Autodesk Inventor part; units mm, degrees
ref_plane "YZ Plane" through (0, 0, 0) normal (1, 0, 0) x (0, 1, 0)
ref_plane "XZ Plane" through (0, 0, 0) normal (0, 1, 0) x (-1, 0, 0)
ref_plane "XY Plane" through (0, 0, 0) normal (0, 0, 1) x (1, 0, 0)
sketch "Эскиз1" plane through (0, 0, 0) normal (0, 1, 0) x (-1, 0, 0)
  circle A0 centre (0, 0) radius 6.95
  circle A1 centre (0, 0) radius 7.95
  line L0 (0, 0) -> (6.3439, 4.7913)
  line L1 (0, 0) -> (6.3439, -4.7913)
  point P0 (5.546, -4.1887)
  point P1 (5.546, 4.1887)
  dimension "d0" = 13.9
  dimension "d1" = 15.9
extrude "Выдавливание1" add sketch "Эскиз1" along normal blind 30 contours A0 L1 A1 L0 picked at (-7.4629, 1.2262)
sketch "Эскиз2" plane through (0, 30, 0) normal (0, 1, 0) x (1, 0, 0)
  arc A0 (-5.546, -4.1887) -> (-6.4386, -3.6588) centre (-8.2473, -7.7226) ccw
  arc A1 (-6.4386, -3.6588) -> (-7.5956, -5.4645) centre (-6.873, -4.654) ccw
  line L0 (-7.5956, -5.4645) -> (-6.9243, -4.6101)
  arc A2 (-6.3454, -4.7768) -> (-6.9243, -4.6101) centre (-6.7137, -4.9672) ccw
  line L1 (-5.546, -4.1887) -> (-6.3439, -4.7913)
  line L2 (-6.3439, -4.7913) -> (-5.546, -4.1887)
  line L3 (-6.3439, -4.7913) -> (-6.3454, -4.7768)
  line L4 (-0.0151, 0) -> (-3.489, 0)
  arc A3 (-6.4386, 3.6588) -> (-5.546, 4.1887) centre (-8.2473, 7.7226) ccw
  arc A4 (-6.9243, 4.6101) -> (-6.3454, 4.7768) centre (-6.7137, 4.9672) ccw
  line L5 (-5.546, 4.1887) -> (-6.3439, 4.7913)
  line L6 (-6.3439, 4.7913) -> (-5.546, 4.1887)
  line L7 (-6.3439, 4.7913) -> (-6.3454, 4.7768)
  arc A5 (-7.5956, 5.4645) -> (-6.4386, 3.6588) centre (-6.873, 4.654) ccw
  line L8 (-7.5956, 5.4645) -> (-6.9243, 4.6101)
  point P0 (-5.546, 4.1887)
  point P1 (-6.3439, -4.7913)
  point P2 (-5.3694, -4.0591)
  point P3 (-6.3439, 4.7913)
  point P4 (-5.3694, 4.0591)
  point P5 (-6.3439, 4.7913)
  dimension "d25" = 1.0859
sketch "Эскиз3" plane through (0, 30, 0) normal (0, 1, 0) x (1, 0, 0)
  arc A0 (-6.3439, -4.7913) -> (-6.3439, 4.7913) centre (0, 0) ccw
  line L0 (11.5, -6.95) -> (11.5, 6.95)
  arc A1 (-5.546, -4.1887) -> (-5.546, 4.1887) centre (0, 0) ccw
  line L1 (0, -7.95) -> (0, -6.95)
  line L2 (0, 6.95) -> (0, 7.95)
  line L3 (11.5, 6.95) -> (11.5, 10.95)
  line L4 (11.5, -6.95) -> (11.5, -10.95)
  line L5 (0, 3.45) -> (0, 7.95)
  line L6 (11.5, -10.95) -> (0, -10.95)
  line L7 (0, -10.95) -> (0, -7.95)
  line L8 (11.5, 10.95) -> (0, 10.95)
  line L9 (0, 10.95) -> (0, 7.95)
  arc A2 (0, -6.95) -> (0, 6.95) centre (0, 0) ccw
  dimension "d13" = 4
  dimension "d14" = 4
  dimension "d22" = 21.9
  dimension "d23" = 4
extrude "Выдавливание3" add sketch "Эскиз3" against normal blind 30
ref_plane "РабПлоскость1" through (11.5, 20, 4.95) normal (1, 0, 0) x (0, 0, -1)
sketch "Эскиз4" plane through (11.5, 20, 4.95) normal (1, 0, 0) x (0, 0, -1)
  line L0 (4.95, -20) -> (4.95, 10)
  line L1 (1, 10) -> (8.9, 10)
  circle A0 centre (4.95, -12) radius 5
  line L2 (14.4, -20) -> (-4.5, -20)
  circle A1 centre (4.95, 2) radius 5
  line L3 (-4.5, 10) -> (14.4, 10)
  point P0 (7.3306, 10)
  point P1 (2.5694, 10)
  point P2 (4.95, 10)
  dimension "d15" = 10
  dimension "d16" = 8
  dimension "d17" = 10
  dimension "d18" = 8
extrude "Выдавливание4" cut sketch "Эскиз4" against normal blind 2
extrude "Выдавливание5" add sketch "Эскиз2" against normal blind 30
sketch "Эскиз5" plane through (0, 30, 0) normal (0, 1, 0) x (1, 0, 0)
  arc A0 (0, 7.95) -> (-6.3439, 4.7913) centre (0, 0) ccw
  line L0 (-6.3439, 4.7913) -> (-6.3454, 4.7768)
  arc A1 (-6.9243, 4.6101) -> (-6.3454, 4.7768) centre (-6.7137, 4.9672) ccw
  line L1 (-6.9243, 4.6101) -> (-7.5956, 5.4645)
  arc A2 (-7.5956, 5.4645) -> (-6.4386, 3.6588) centre (-6.873, 4.654) ccw
  arc A3 (-6.4386, 3.6588) -> (-5.546, 4.1887) centre (-8.2473, 7.7226) ccw
  arc A4 (-5.546, -4.1887) -> (-5.546, 4.1887) centre (0, 0) ccw
  arc A5 (-5.546, -4.1887) -> (-6.4386, -3.6588) centre (-8.2473, -7.7226) ccw
  arc A6 (-6.4386, -3.6588) -> (-7.5956, -5.4645) centre (-6.873, -4.654) ccw
  line L2 (-7.5956, -5.4645) -> (-6.9243, -4.6101)
  arc A7 (-6.3454, -4.7768) -> (-6.9243, -4.6101) centre (-6.7137, -4.9672) ccw
  line L3 (-6.3454, -4.7768) -> (-6.3439, -4.7913)
  arc A8 (-6.3439, -4.7913) -> (0, -7.95) centre (0, 0) ccw
  line L4 (0, -7.95) -> (0, -10.95)
  line L5 (0, -10.95) -> (11.5, -10.95)
  line L6 (11.5, -10.95) -> (11.5, 10.95)
  line L7 (11.5, 10.95) -> (0, 10.95)
  line L8 (0, 10.95) -> (0, 7.95)
  line L9 (0, 6.95) -> (0, 7.95)
  line L10 (0, -6.95) -> (0, -7.95)
extrude "Выдавливание6" [suppressed]
sketch "Эскиз6" plane through (11.5, 30, 10.95) normal (1, 0, 0) x (0, 0, -1)
  arc A0 (15.95, -22) -> (15.95, -22) centre (10.95, -22) ccw
  arc A1 (15.95, -8) -> (15.95, -8) centre (10.95, -8) ccw
  point P0 (10.95, -30)
extrude "Выдавливание7" [suppressed]
properties part number "крепление маркера 14мм"
The listing builds one solid part. Answer for the finished solid, in the listing's coordinates (mm). A direction names the side the tool comes from. Coordinates: 2 decimals unless noted, no trailing zeros. Loops run counter-clockwise (first coordinate to the right, second up) from the corner with the lowest first, then second, coordinate; pieces in that order, holes last. Notation, with made-up numbers: M -28.75,59 L 23.25,59 A18 ccw 23.25,81 Z; hole C 30,27.25 d11. An arc over 180 degrees is marked long. Answer as CSV lines item,"result". Start each with the question number.
(1) Find the intervals of material crossed by L1, parallel to Y at x = 10.5, z = 0; L2, parallel to Z at x = 10.55, y = 22; L3, parallel to X at y = 24.25, z = 5, in increasing order. Write a range as [from, to].
(2) Given pin 1 (1 mm diameter, centred on y = 24, z = 1, fed in from -X); pin 2 (1.5 mm diameter, centred on y = 15.5, z = -9, fed in from -X); pin 3 (1.5 mm diameter, centred on x = -1.5, y = 18.5, fed in from -Z), each flat-ended and moving along its own axis, determine where each tip first touches the part or whether it passes through.
(3) The mould has two halves that part along Y. Classify faces 1 (the cylindrical face through (-7.8, 15.21, -4.09)), 2 (the flat face through (9.5, 22, 0)), 3 (the flat face through (8, 0, 0)): pulls with the +Y half, pulls with the -Y half, needs draft (parallel to the pull), parting line crosses it, or undercut.
(4) The part is cut by section A-A (x = 5.25). Give the vertices of the cut face in (y, z), and give its area (3 significant figures).
(5) The part is cut by section D-D (z = -6.5). Give the vertices of the cut face in (x, y), and give its area (3 significant figures).
(6) For faces 4 (the flat face through (0, 15, -9)), 5 (the flat face through (-7.26, 15.21, -5.04)), 6 (the flat face through (0, 15, 9)), 7 (the cylindrical face through (10.51, 17.12, 1.08)), 8 (the cylindrical face through (-5.97, 15.21, 3.9)), determine the directions among +Z, -Z, +X, -X, +Y, -Y from which every point of the face is accessible in a straight line to the end or side of a thin tool.
(7) The part is cut by section B-B (z = 0). Give the vertices of the cut face in (x, y).
Determined:
1,L1,"[0, 3], [13, 17], [27, 30]"
1,L2,"[-10.95, -5], [5, 10.95]"
1,L3,"[-7.9, -7.23], [-6.18, -4.83], [4.83, 11.5]"
2,pin 1,"x = 6.79"
2,pin 2,"x = 0"
2,pin 3,"z = -7.91"
3,face 1,"needs draft"
3,face 2,"undercut"
3,face 3,"pulls with the -Y half"
4,outline,"M 0,-10.95 L 30,-10.95 L 30,-4.55 L 0,-4.55 Z; M 0,4.55 L 30,4.55 L 30,10.95 L 0,10.95 Z"
4,area,"384 mm2"
5,outline,"M -4.58,0 L -2.46,0 L -2.46,30 L -4.58,30 Z; M 2.46,0 L 11.5,0 L 11.5,30 L 2.46,30 Z"
5,area,"335 mm2"
6,face 4,"-Z, -X, +Y, -Y"
6,face 5,"-Z, +Y, -Y"
6,face 6,"+Z, -X, +Y, -Y"
6,face 7,"+X"
6,face 8,"+Y, -Y"
7,outline,"M 6.95,0 L 11.5,0 L 11.5,3 L 9.5,3 L 9.5,13 L 11.5,13 L 11.5,17 L 9.5,17 L 9.5,27 L 11.5,27 L 11.5,30 L 6.95,30 Z"
